Input: part model. Units: mm. Frame: model coordinates. Face numbers are marked on the shaded views. A direction names the side the tool comes from. Give positions to 0.01 mm unless a question says otherwise; leave off trailing zeros. Loops run counter-clockwise (first coordinate to the right, second up) from the corner with the lowest first, then second, coordinate; pieces in that order, holes last.
from build123d import *


with BuildPart() as part:
    # Esquisse1 → Révolution1 (revolve)
    with BuildSketch(Plane.XY):
        with BuildLine():
            Line((-7, 0), (-7, 1))
            Line((-7, 1), (-5.51771325, 1))
            ThreePointArc((-5.51771325, 1), (-4.660362956, 1.211647907), (-4, 1.79796278))
            ThreePointArc((-4, 1.79796278), (-2.634488917, 1.648039478), (-1.334035601, 1.205412449))
            ThreePointArc((-1.334035601, 1.205412449), (0, 1.79796278), (1.334035601, 1.205412449))
            ThreePointArc((1.334035601, 1.205412449), (2.634488917, 1.648039478), (4, 1.79796278))
            ThreePointArc((4, 1.79796278), (4.660362956, 1.211647907), (5.51771325, 1))
            Line((5.51771325, 1), (7, 1))
            Line((7, 1), (7, 0))
            Line((7, 0), (-7, 0))
        make_face()
    revolve(axis=Axis((-7, 0, 0), (1, 0, 0)))


solid = part.part
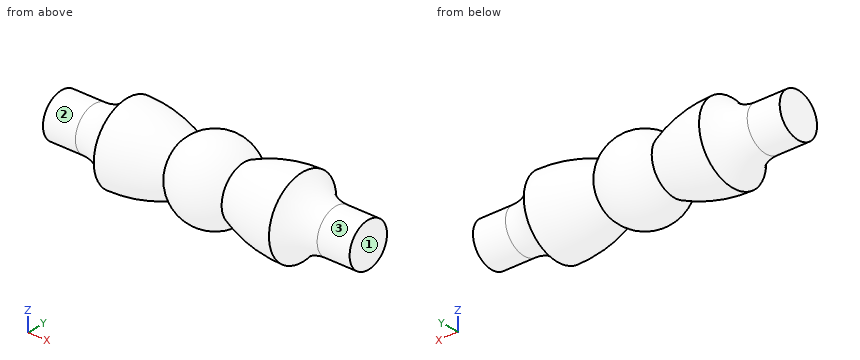
(1) Pin query (flat end, axial travel): pin 1 Ø1.5 at (x, y) = (-2.5, -0.5) entering from -Z. Return the tip coordinate at first contact, or that it passes through.
Values follow:
pin 1: stops at z = -1.74
(2) Reachability of the marked faces 1, 2 and 3 from +Z, -Z, +X, -X, +Y, -Y: full face, straight path, thin tool, end or side. Return the list, or none.
Values follow:
face 1: +Z, -Z, +X, +Y, -Y
face 2: -X
face 3: +X
(3) Ray query, probe 1 along Y at (x, z) = (-0.75, 0.9); probe 2 along Z at (x, y) = (-0.5, 0.9); probe 3 along Y at (x, z) = (2, 1.1). Return the intervals inside material, ascending.
Values follow:
probe 1: y = -1.36 to 1.36
probe 2: z = -1.47 to 1.47
probe 3: y = -0.98 to 0.98
(4) Cut plane A-A (x = 0.5). Return the cut outline in (y, z), and give its area (3 significant figures).
Values follow:
outline: circle Ø3.45 at (0, 0)
area: 9.37 mm2
